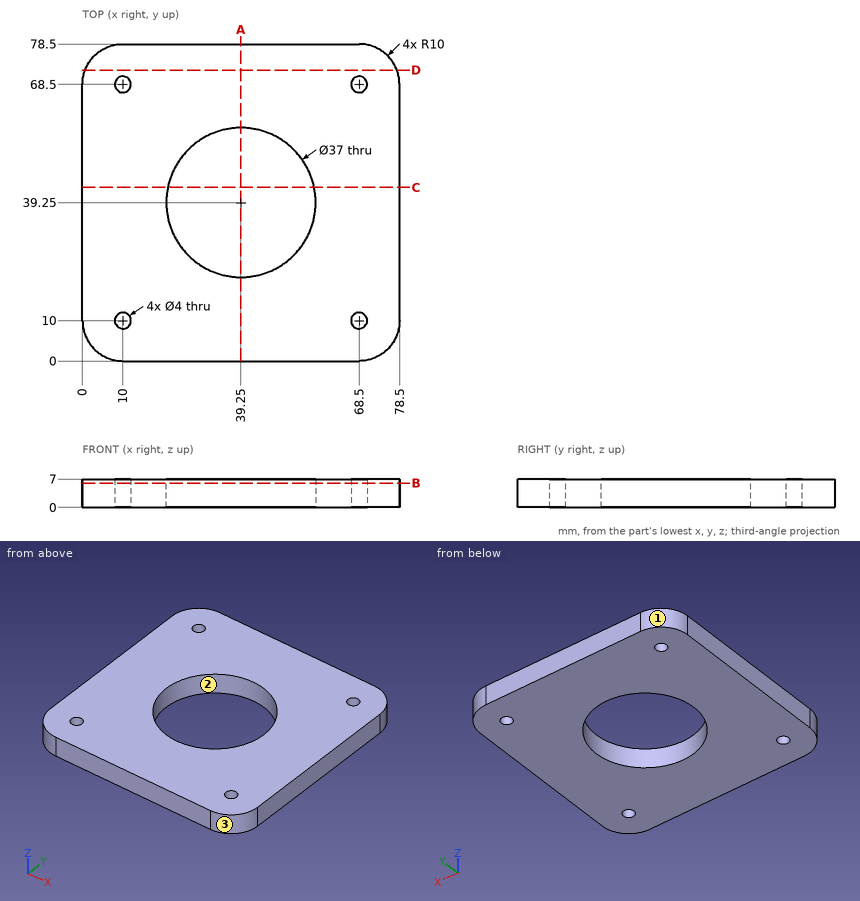
Verification items for this drawing (mm, ordinates from the low corner). Give positions to 0.01 mm unless a question says otherwise; leave off trailing zeros. Loops run counter-clockwise (first coordinate to the right, second up) from the corner with the lowest first, then second, coordinate; pieces in that order, holes last. Notation, with made-up numbers: M -12,-24.5 L 24,-24.5 A21 ccw 24,-13.5 Z; hole C 84.25,56.25 d9. An arc over 180 degrees is marked long. Answer in a Markdown table with one row per item.
1) Depth check by flat-ended pin: pin 1 (2.5 mm diameter, centred on x = 10, y = 10, fed in from -Z). Enter the tip coordinate at first touch or a pass-through.
Solutions:
| item | result |
|---|---|
| pin 1 | passes through |
2) Cross-section at D-D (y = 72). Enter the section's corners in (x, z), plus the area to 3 significant figures.
Solutions:
| item | result |
|---|---|
| outline | M 0.63,0 L 77.87,0 L 77.87,7 L 0.63,7 Z |
| area | 541 mm^2 |
3) Cross-section at A-A (x = 39.25). Enter the section's corners in (y, z), plus the area to 4 significant figures.
Solutions:
| item | result |
|---|---|
| outline | M 0,0 L 20.75,0 L 20.75,7 L 0,7 Z; M 57.75,0 L 78.5,0 L 78.5,7 L 57.75,7 Z |
| area | 290.5 mm^2 |
4) Cross-section at C-C (y = 43). Enter the section's corners in (x, z).
Solutions:
| item | result |
|---|---|
| outline | M 0,0 L 21.13,0 L 21.13,7 L 0,7 Z; M 57.37,0 L 78.5,0 L 78.5,7 L 57.37,7 Z |
5) Cross-section at B-B (z = 6). Enter the section's corners in (x, y), plus the area to 3 significant figures.
Solutions:
| item | result |
|---|---|
| outline | M 0,10 A10 ccw 10,0 L 68.5,0 A10 ccw 78.5,10 L 78.5,68.5 A10 ccw 68.5,78.5 L 10,78.5 A10 ccw 0,68.5 Z; hole C 10,10 d4; hole C 10,68.5 d4; hole C 39.25,39.25 d37; hole C 68.5,10 d4; hole C 68.5,68.5 d4 |
| area | 4,950 mm^2 |
6) Thickness scan on line 1 (X direction, y = 68.5, z = 2.5); line 2 (Y direction, x = 67.5, z = 3.75). Record the ranges inside material, lowest first.
Solutions:
| item | result |
|---|---|
| line 1 | x = 0 to 8, 12 to 66.5, 70.5 to 78.5 |
| line 2 | y = 0 to 8.27, 11.73 to 66.77, 70.23 to 78.5 |
7) Mould release check, pull along X, two halves, no side actions. Record for the marked faces 1, 2 and 3: released by +X, released by -X, zero draft, split by the parting line, or undercut.
Solutions:
| item | result |
|---|---|
| face 1 | released by -X |
| face 2 | undercut |
| face 3 | released by +X |
